Source: CAD feature listing. Evaluate the final solid. Frame: model axes, mm. Face numbers are marked on the shaded views. Give positions to 0.01 mm unless a question says otherwise; leave off trailing zeros. Write each loop counter-clockwise with the first axis right and the second up, starting at its lowest first coordinate (ties: lowest second). Pieces come first, ordered by that corner, then holes. Notation, with made-up numbers: (56, 8.25) -> (71, 8.25) arc R23 ccw to (71, 16.25) -> close; hole circle Ø1 at (-31, 62). An arc over 180 degrees is marked (long way). Write item = value, one per line.
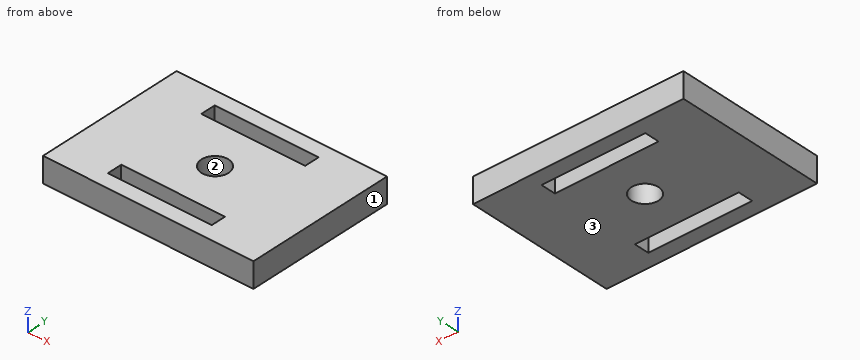
Autodesk Inventor part; units mm, degrees
ref_plane "YZ Plane" through (0, 0, 0) normal (1, 0, 0) x (0, 1, 0)
ref_plane "XZ Plane" through (0, 0, 0) normal (0, 1, 0) x (-1, 0, 0)
ref_plane "XY Plane" through (0, 0, 0) normal (0, 0, 1) x (1, 0, 0)
sketch "Эскиз1" plane through (0, 0, 0) normal (0, 0, 1) x (1, 0, 0)
  line L0 (-21, -15) -> (21, -15)
  line L1 (21, -15) -> (21, 15)
  line L2 (21, 15) -> (-21, 15)
  line L3 (-21, 15) -> (-21, -15)
  line L4 (-21, -15) -> (21, 15) construction
  line L5 (21, -15) -> (-21, 15) construction
  circle A0 centre (0, 0) radius 2.7
  line L6 (-10.7143, 15) -> (-10.7143, 12) construction
  line L7 (10.7143, 15) -> (10.7143, 13) construction
  line L8 (-10.7143, 12) -> (10, 12)
  line L9 (10, 12) -> (10, 9)
  line L10 (10, 9) -> (-10.7143, 9)
  line L11 (-10.7143, 9) -> (-10.7143, 12)
  line L12 (-21, 0) -> (21, 0) construction
  line L13 (-10.7143, -12) -> (10, -12)
  line L14 (10, -12) -> (10, -9)
  line L15 (-10.7143, -9) -> (-10.7143, -12)
  line L16 (10, -9) -> (-10.7143, -9)
  dimension "d0" = 42
  dimension "d1" = 30
  dimension "d2" = 5.4
  dimension "d3" = 3
  dimension "d4" = 2
  dimension "d5" = 3
extrude "Выдавливание1" add sketch "Эскиз1" along normal blind 5
properties part number "Female for pack"
1) Cut plane B-B (y = 0). Return the cut outline in (x, z).
Computed:
outline = (-21, 0) -> (-2.7, 0) -> (-2.7, 5) -> (-21, 5) -> close; (2.7, 0) -> (21, 0) -> (21, 5) -> (2.7, 5) -> close
2) Draft query along X for the marked faces 1, 2 and 3. Return one class per face: pulls with the +X half, pulls with the -X half, needs draft (parallel to the pull), parting line crosses it, or undercut.
Computed:
face_1 = pulls with the +X half
face_2 = undercut
face_3 = needs draft
3) Cut plane D-D (y = -10.5). Return the cut outline in (x, z), then the cut area to 3 significant figures.
Computed:
outline = (-21, 0) -> (-10.71, 0) -> (-10.71, 5) -> (-21, 5) -> close; (10, 0) -> (21, 0) -> (21, 5) -> (10, 5) -> close
area = 106 mm²
4) Material intervals for L1, parallel to Y at x = 9.5, z = 1.5; L2, parallel to Y at x = 0, z = 2.3; L3, parallel to X at y = -9.5, z = 2.8, sorted ascending.
Computed:
L1 = -15 to -12, -9 to 9, 12 to 15
L2 = -15 to -12, -9 to -2.7, 2.7 to 9, 12 to 15
L3 = -21 to -10.71, 10 to 21
5) Cut plane C-C (z = 3.75). Return the cut outline in (x, y), then the cut area to 3 significant figures.
Computed:
outline = (-21, -15) -> (21, -15) -> (21, 15) -> (-21, 15) -> close; hole (-10.71, -12) -> (10, -12) -> (10, -9) -> (-10.71, -9) -> close; hole (-10.71, 9) -> (10, 9) -> (10, 12) -> (-10.71, 12) -> close; hole circle Ø5.4 at (0, 0)
area = 1,110 mm²
6) Cut plane A-A (x = 4). Return the cut outline in (y, z), then the cut area to 3 significant figures.
Computed:
outline = (-15, 0) -> (-12, 0) -> (-12, 5) -> (-15, 5) -> close; (-9, 0) -> (9, 0) -> (9, 5) -> (-9, 5) -> close; (12, 0) -> (15, 0) -> (15, 5) -> (12, 5) -> close
area = 120 mm²
7) Contact query for flat-ended pins moving along their axis: pin 1 (4.5 mm diameter, centred on x = 0, y = 0, fed in from -Z); pin 2 (1 mm diameter, centred on x = -8.5, y = -3, fed in from -Z). Output: stop coordinate, or through.
Computed:
pin_1 = through
pin_2 = 0
